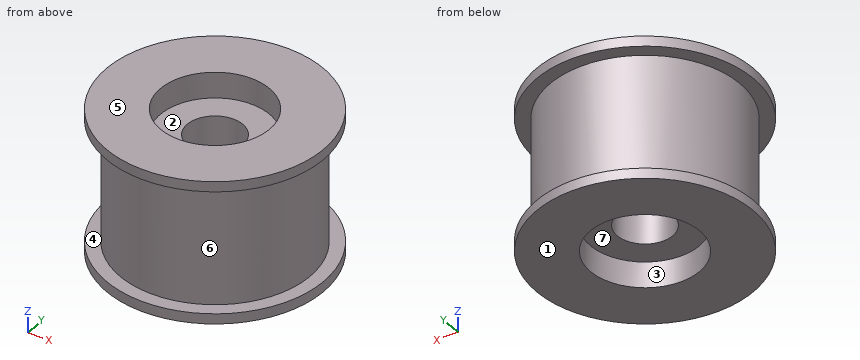
from build123d import *

# Parameters (mm, degrees)
SKETCH1_R           = 14
SKETCH1_R_2         = 4.1
BOSS_EXTRUDE1_DEPTH = 21
SKETCH8_R           = 16
SKETCH8_R_2         = 6.25
BOSS_EXTRUDE2_DEPTH = 1.5
SKETCH9_R           = 16
SKETCH9_R_2         = 6.25
BOSS_EXTRUDE3_DEPTH = 1.5
SKETCH10_R          = 8.05
CUT_EXTRUDE1_DEPTH  = 3.8
CUT_EXTRUDE2_START  = -21
SKETCH10_2_R        = 8.05
CUT_EXTRUDE2_DEPTH  = 3.8


with BuildPart() as part:
    # Sketch1 → Boss-Extrude1 (new body)
    with BuildSketch(Plane.XY):
        Circle(SKETCH1_R)
        Circle(SKETCH1_R_2, mode=Mode.SUBTRACT)
    extrude(amount=BOSS_EXTRUDE1_DEPTH)

    # Sketch8 → Boss-Extrude2 (add)
    with BuildSketch(Plane(origin=(0, 0, 21), x_dir=(-1, 0, 0), z_dir=(0, 0, -1))):
        Circle(SKETCH8_R)
        Circle(SKETCH8_R_2, mode=Mode.SUBTRACT)
    extrude(amount=BOSS_EXTRUDE2_DEPTH)

    # Sketch9 → Boss-Extrude3 (add)
    with BuildSketch(Plane.XY):
        Circle(SKETCH9_R)
        Circle(SKETCH9_R_2, mode=Mode.SUBTRACT)
    extrude(amount=BOSS_EXTRUDE3_DEPTH)

    # Sketch10 → Cut-Extrude1 (cut)
    with BuildSketch(Plane.XY.offset(21)):
        Circle(SKETCH10_R)
    extrude(amount=-CUT_EXTRUDE1_DEPTH, mode=Mode.SUBTRACT)

    # Sketch10<2> → Cut-Extrude2 (cut)
    with BuildSketch(Plane.XY.offset(21).offset(CUT_EXTRUDE2_START)):
        Circle(SKETCH10_2_R)
    extrude(amount=CUT_EXTRUDE2_DEPTH, mode=Mode.SUBTRACT)


solid = part.part
The listing builds one solid part. Answer for the finished solid, in the listing's coordinates (mm). Face numbers are marked on the shaded views. A direction names the side the tool comes from. Coordinates: 2 decimals unless noted, no trailing zeros. Write each loop counter-clockwise with the first axis right and the second up, starting at its lowest first coordinate (ties: lowest second). Pieces come first, ordered by that corner, then holes. Notation, with made-up numbers: M 74.5,46 L 126.5,46 A20 ccw 126.5,68 Z; hole C -29.5,77 d10. An arc over 180 degrees is marked long. Put each result on its own line as item: value. Start each with the question number.
1. Which of the six approach directions +Z, -Z, +X, -X, +Y, -Y give full straight-line access (tool end or side, diameter ignored) to the marked faces 1, 2, 3 and 4?
2. For a pull along Y with two mould halves and no side action, classify the marked faces 5, 6 and 7 as pulls with the +Y half, pulls with the -Y half, needs draft (parallel to the pull), parting line crosses it, or undercut.
3. A cutting plane is placed at D-D on x = -6.5. Write down the section's boundary in (y, z), then the cut area to 3 significant figures.
4. A cutting plane is placed at C-C on z = 13. Write down the section's boundary in (x, y).
5. Consider line 1 (Y direction, x = 0, z = 18.3); line 2 (Y direction, x = 0, z = 19.7); line 3 (X direction, y = 0, z = 10). Determine where each line is inside the solid, lowest interval first. Write a range as from..to.
6. A cutting plane is placed at A-A on y = 0. Write down the section's boundary in (x, z).
7. Flat-ended cylindrical pins translate along their axes: P1, Ø9.5, axis at x = 0, y = 0, coming from the +Z side; P2, Ø16, axis at x = 0, y = -7, coming from the +Z side; P3, Ø10, axis at x = 1, y = 2, coming from the -Z side; P4, Ø1, axis at x = 4.5, z = 9, coming from the +Y side. Find the tip coordinate at first contact, or state that the pin passes through.
Resolved:
1. face 1: -Z, +X, -X, +Y, -Y
1. face 2: +Z
1. face 3: -Z
1. face 4: none
2. face 5: needs draft
2. face 6: parting line crosses it
2. face 7: undercut
3. outline: M -14.62,0 L -4.75,0 L -4.75,3.8 L 4.75,3.8 L 4.75,0 L 14.62,0 L 14.62,1.5 L 12.4,1.5 L 12.4,19.5 L 14.62,19.5 L 14.62,21 L 4.75,21 L 4.75,17.2 L -4.75,17.2 L -4.75,21 L -14.62,21 L -14.62,19.5 L -12.4,19.5 L -12.4,1.5 L -14.62,1.5 Z
3. area: 462 mm2
4. outline: C 0,0 d28; hole C 0,0 d8.2
5. line 1: y = -14..-8.05, 8.05..14
5. line 2: y = -16..-8.05, 8.05..16
5. line 3: x = -14..-4.1, 4.1..14
6. outline: M -16,0 L -8.05,0 L -8.05,3.8 L -4.1,3.8 L -4.1,17.2 L -8.05,17.2 L -8.05,21 L -16,21 L -16,19.5 L -14,19.5 L -14,1.5 L -16,1.5 Z; M 4.1,3.8 L 8.05,3.8 L 8.05,0 L 16,0 L 16,1.5 L 14,1.5 L 14,19.5 L 16,19.5 L 16,21 L 8.05,21 L 8.05,17.2 L 4.1,17.2 Z
7. P1: stops at z = 17.2
7. P2: stops at z = 21
7. P3: stops at z = 3.8
7. P4: stops at y = 13.42
